Design review of the part shown in the three views and the two pictorial views. Dimensions are in mm from the part's minimum x, y and z. A direction names the side the tool comes from. Round coordinates to 2 decimals unless told otherwise and drop trailing zeros. Loops run counter-clockwise (first coordinate to the right, second up) from the corner with the lowest first, then second, coordinate; pieces in that order, holes last.
1) Take a section at A-A (x = 64). State the section outline as (y, z) points, then the cut area to 3 significant figures.
2) Take a section at D-D (z = 68.5). State the section outline as (x, y) points, then the cut area to 3 significant figures.
3) Mouldability with a two-part tool opening along Y and no side actions: class the marked faces 3, 4 and 5 as pulls with the +Y half, pulls with the -Y half, needs draft (parallel to the pull), parting line crosses it, or undercut.
4) Tool access review of the marked faces 1 and 2: name each direction out of +Z, -Z, +X, -X, +Y, -Y from which nothing blocks a thin tool from reaching the whole face with its end or side.
5) Take a section at C-C (y = 40.5). State the section outline as (x, z) points, then the cut area to 3 significant figures.
6) Take a section at B-B (z = 83). State the section outline as (x, y) points.
7) Wall thickness on L1, parallel to Y at x = 46, z = 92; L2, parallel to X at y = 5, z = 61.5: over which ranges is each line inside the solid? List them lowest first.
8) Insertion check: pin 1 (12 mm diameter, centred on y = 12.5, z = 56, fed in from +X). The pin has a flat end and moves straight along its axis. Give the tip position at first contact, or say it passes through.
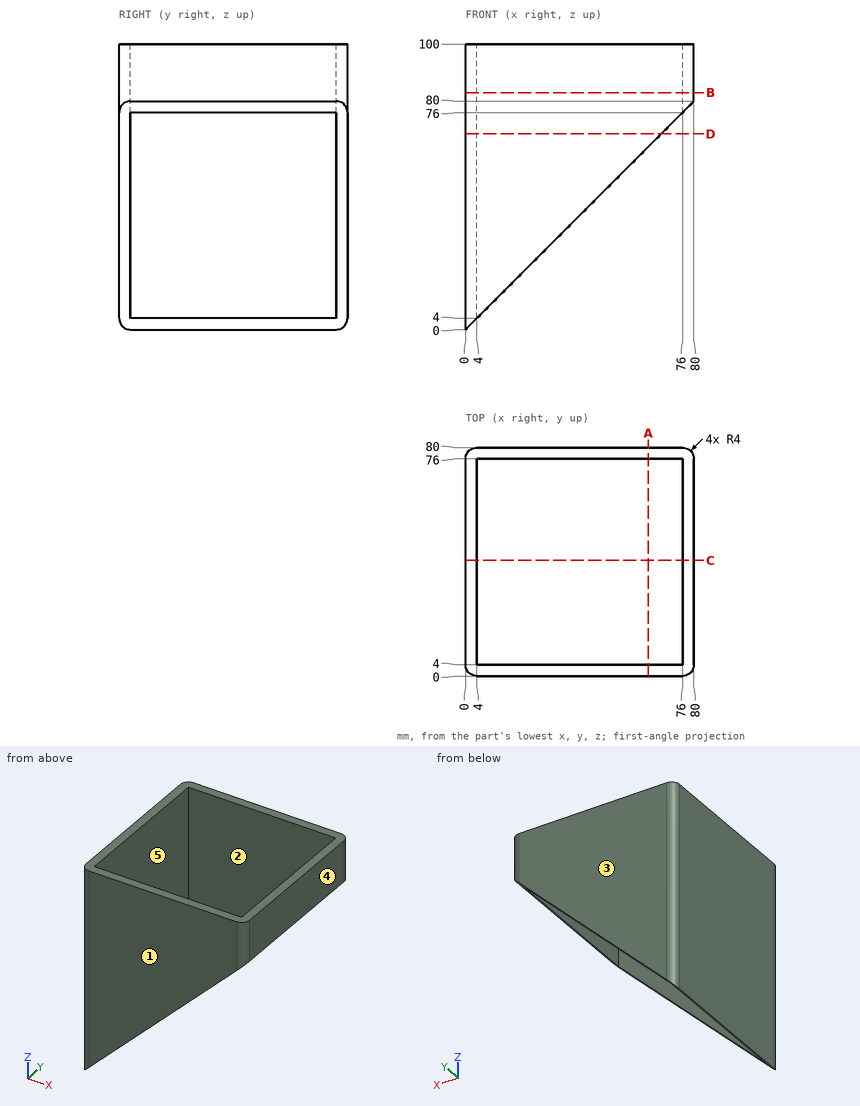
Response:
1. outline: (0, 64) - (4, 64) - (4, 100) - (0, 100) - close; (76, 64) - (80, 64) - (80, 100) - (76, 100) - close
1. area: 288 mm2
2. outline: (0, 4) arc R4 ccw to (4, 0) - (68.5, 0) - (68.5, 4) - (4, 4) - (4, 76) - (68.5, 76) - (68.5, 80) - (4, 80) arc R4 ccw to (0, 76) - close
2. area: 829 mm2
3. face 3: pulls with the +Y half
3. face 4: needs draft
3. face 5: undercut
4. face 1: +Z, -Z, +X, -X, -Y
4. face 2: +Z, -Z
5. outline: (0, 0) - (4, 4) - (4, 100) - (0, 100) - close; (76, 76) - (80, 80) - (80, 100) - (76, 100) - close
5. area: 480 mm2
6. outline: (0, 4) arc R4 ccw to (4, 0) - (76, 0) arc R4 ccw to (80, 4) - (80, 76) arc R4 ccw to (76, 80) - (4, 80) arc R4 ccw to (0, 76) - close; hole (4, 4) - (76, 4) - (76, 76) - (4, 76) - close
7. L1: y = 0 to 4, 76 to 80
7. L2: x = 0 to 4
8. pin 1: stops at x = 4
